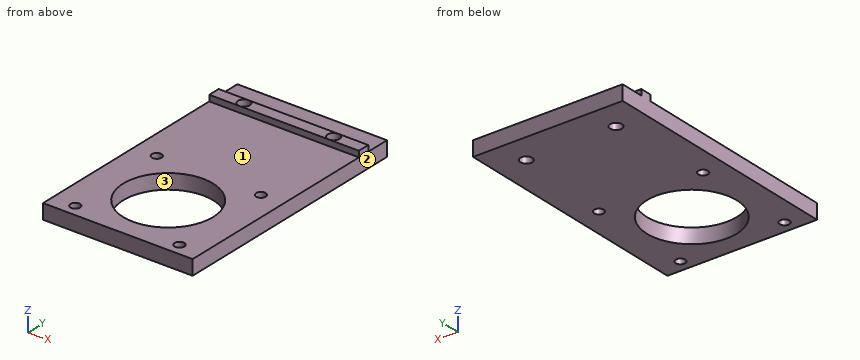
Autodesk Inventor part; units mm, degrees
ref_plane "YZ Plane" through (0, 0, 0) normal (1, 0, 0) x (0, 1, 0)
ref_plane "XZ Plane" through (0, 0, 0) normal (0, 1, 0) x (-1, 0, 0)
ref_plane "XY Plane" through (0, 0, 0) normal (0, 0, 1) x (1, 0, 0)
sketch "Sketch1" plane through (0, 0, 0) normal (0, 0, 1) x (1, 0, 0)
  line L0 (0, 116.2) -> (0, -116.2)
  line L1 (-70, 0) -> (70, 0)
  line L2 (-50, -83) -> (50, -83)
  line L3 (50, -83) -> (50, 83)
  line L4 (50, 83) -> (-50, 83)
  line L5 (-50, 83) -> (-50, -83)
  circle A0 centre (0, -40) radius 30
  circle A1 centre (-30, 63) radius 4
  circle A2 centre (30, 63) radius 4
  circle A3 centre (34.8, -74.8) radius 3.25
  circle A4 centre (34.8, -5.2) radius 3.25
  circle A5 centre (-34.8, -5.2) radius 3.25
  circle A6 centre (-34.8, -74.8) radius 3.25
  line L6 (-30, 63) -> (-30, 59)
  line L7 (0, -40) -> (0, -10)
  point P0 (0, 0)
  dimension "d2" = 60
  dimension "d4" = 8
  dimension "d0" = 100
  dimension "d1" = 166
  dimension "d3" = 43
  dimension "d5" = 8
  dimension "d6" = 20
  dimension "d7" = 20
  dimension "d8" = 20
  dimension "d9" = 20
  dimension "d10" = 6.5
  dimension "d11" = 6.5
  dimension "d12" = 6.5
  dimension "d13" = 6.5
  dimension "d14" = 69.6
  dimension "d15" = 69.6
  dimension "d16" = 69.6
  dimension "d17" = 69.6
  dimension "d18" = 0
  dimension "d19" = 0
  dimension "d20" = 34.8
  dimension "d21" = 34.8
  dimension "d22" = 69
extrude "Extrusion1" add sketch "Sketch1" along normal blind 20 contours A0 L0 L2 L5 L1 | L0 L1 L3 L2 A0 | L1 L5 L4 L0 | L0 L4 L3 L1
sketch "Sketch2" plane through (0, 0, 20) normal (0, 0, 1) x (1, 0, 0)
  line L0 (50, 83) -> (-50, 83)
  line L1 (-50, 83) -> (-50, -83)
  line L2 (-50, -83) -> (50, -83)
  line L3 (50, -83) -> (50, 83)
  circle A0 centre (30, 63) radius 4
  circle A1 centre (34.8, -5.2) radius 3.25
  circle A2 centre (34.8, -74.8) radius 3.25
  circle A3 centre (-34.8, -74.8) radius 3.25
  circle A4 centre (-34.8, -5.2) radius 3.25
  circle A5 centre (-30, 63) radius 4
  circle A6 centre (0, -40) radius 30
  line L4 (-50, 83) -> (-50, -83)
  line L5 (-50, 63) -> (50, 63)
  line L6 (-50, 67) -> (50, 67)
  line L7 (-50, 59) -> (50, 59)
  point P0 (0, 0)
  point P1 (50, 59)
  point P2 (-50, 59)
  point P3 (-50, 67)
  point P4 (50, 67)
  dimension "d25" = 4
  dimension "d26" = 4
extrude "Extrusion2" cut sketch "Sketch2" against normal blind 4 contours L3 L6 L1 L0 | L3 L2 L1 L7
sketch "Sketch3" plane through (0, 0, 0) normal (0, 0, -1) x (-1, 0, 0)
  line L0 (-50, 83) -> (50, 83)
  line L1 (-50, -83) -> (-50, 83)
  line L2 (50, -83) -> (-50, -83)
  line L3 (50, 83) -> (50, -83)
  circle A0 centre (-30, 63) radius 4
  circle A1 centre (-34.8, -5.2) radius 3.25
  circle A2 centre (-34.8, -74.8) radius 3.25
  circle A3 centre (34.8, -74.8) radius 3.25
  circle A4 centre (34.8, -5.2) radius 3.25
  circle A5 centre (30, 63) radius 4
  circle A6 centre (0, -40) radius 30
  point P0 (0, 0)
extrude "Extrusion3" cut sketch "Sketch3" against normal blind 6
properties part number "motor mount middle"
The listing builds one solid part. Answer for the finished solid, in the listing's coordinates (mm). Face numbers are marked on the shaded views. Coordinates: 2 decimals unless noted, no trailing zeros. Order: outer loops, then holes, each group sorted by start corner. A loop starts at its lowest first (then second) coordinate and runs counter-clockwise, first axis right, second up. Notation, with made-up numbers: M 62,39.25 L 68,39.25 A13 ccw 68,59.25 Z; hole C 47.25,-31 d5. An arc over 180 degrees is marked long. Answer as a JSON object with one key per item and string values. Group by question number.
1. Determine the mould class of the marked faces 1, 2 and 3 for opening direction X: released by +X, released by -X, zero draft, split by the parting line, or undercut.
2. Straight lines are drawn through the part: line 1 (X direction, y = 63, z = 9); line 2 (Y direction, x = -34.8, z = 13.5); line 3 (Y direction, x = -1.5, z = 17.5). For each, find the intervals that lie inside material, in ascending order.
3. Section D-D on y = -13 is taken. Write down the section's boundary in (x, z).
4. Section B-B on z = 9 is taken. Write down the section's boundary in (x, y).
5. Flat-ended cylindrical pins translate along their axes: P1, Ø3, axis at x = 14.5, y = 38, coming from the +Z side; P2, Ø1.2, axis at x = -24, z = 18.5, coming from the -Y side; P3, Ø7.5, axis at x = -34.8, y = -5.2, coming from the -Z side; P4, Ø1.2, axis at x = -16, z = 17.5, coming from the +Y side. Find the tip coordinate at first contact, or state that the pin passes through.
6. Section C-C on x = -24 is taken. Write down the section's boundary in (y, z).
7. Section A-A on y = -74.8 is taken. Write down the section's boundary in (x, z).
Values follow:
{
 "1": {"face 1": "zero draft", "face 2": "released by +X", "face 3": "undercut"},
 "2": {"line 1": "-50 to -34, -26 to 26, 34 to 50", "line 2": "-83 to -78.05, -71.55 to -8.45, -1.95 to 83", "line 3": "59 to 67"},
 "3": {"outline": "M -50,6 L -13.08,6 L -13.08,16 L -50,16 Z; M 13.08,6 L 50,6 L 50,16 L 13.08,16 Z"},
 "4": {"outline": "M -50,-83 L 50,-83 L 50,83 L -50,83 Z; hole C -34.8,-74.8 d6.5; hole C -34.8,-5.2 d6.5; hole C -30,63 d8; hole C 0,-40 d60; hole C 30,63 d8; hole C 34.8,-74.8 d6.5; hole C 34.8,-5.2 d6.5"},
 "5": {"P1": "z = 16", "P2": "y = 59", "P3": "z = 6", "P4": "y = 67"},
 "6": {"outline": "M -83,6 L -58,6 L -58,16 L -83,16 Z; M -22,6 L 83,6 L 83,16 L 67,16 L 67,20 L 59,20 L 59,16 L -22,16 Z"},
 "7": {"outline": "M -50,6 L -38.05,6 L -38.05,16 L -50,16 Z; M -31.55,6 L 31.55,6 L 31.55,16 L -31.55,16 Z; M 38.05,6 L 50,6 L 50,16 L 38.05,16 Z"}
}
